Build history of the part. All positions in model axes, mm. Give positions to 0.01 mm unless a question says otherwise; leave off trailing zeros. Loops run counter-clockwise (first coordinate to the right, second up) from the corner with the lowest first, then second, coordinate; pieces in that order, holes last. Notation, with made-up numbers: M 63.25,62.5 L 100.25,62.5 A11 ccw 100.25,72.5 Z; hole C 63.5,86.5 d6. An arc over 180 degrees is marked long. Answer as a JSON object with one key per item and string values. Group by question number.
1. Drill centre lines: line 1 along X through (y, z) = (10.1, 27); line 2 along X through (y, z) = (12, 64). Where is each one in solid material? Low to high. Write a range as [from, to].
2. Slice it at B-B (y = 11.3). List the corners of the cut face in (x, z) (3 decimals).
3. Slice it at A-A (z = 22). List the corners of the cut face in (x, y), then the cut area to 3 significant figures.
4. Slice it at C-C (z = 61.5). List the corners of the cut face in (x, y), then the cut area to 4 significant figures.
5. Drop flat-ended pins along their axis: pin 1 Ø1.5 at (x, y) = (9.5, 10.5) entering from +Z; pin 2 Ø1.5 at (x, y) = (10, 10.5) entering from -Z. Give the stop position or say it passes through.
from build123d import *

# Parameters (mm, degrees)
BOX021_W     = 4.2
BOX021_H     = 6
BOX021_DEPTH = 15
BOX020_W     = 4.2
BOX020_H     = 6
BOX020_DEPTH = 15
BOX019_W     = 4.2
BOX019_H     = 6
BOX019_DEPTH = 15
BOX018_W     = 4.2
BOX018_H     = 6
BOX018_DEPTH = 15
BOX017_W     = 10
BOX017_H     = 10
BOX017_DEPTH = 32.4
BOX016_W     = 214
BOX016_H     = 3
BOX016_DEPTH = 96.05
FILLET001_R  = 6


with BuildPart() as obj1:
    # Box021 → Box021 (new body)
    with BuildSketch(Plane(origin=(211.4, 8, 15.25), x_dir=(1, 0, 0), z_dir=(0, 0, 1))):
        with Locations((2.1, 3)):
            Rectangle(BOX021_W, BOX021_H)
    extrude(amount=BOX021_DEPTH)


with BuildPart() as obj2:
    # Box020 → Box020 (new body)
    with BuildSketch(Plane(origin=(8.4, 8, 15.25), x_dir=(1, 0, 0), z_dir=(0, 0, 1))):
        with Locations((2.1, 3)):
            Rectangle(BOX020_W, BOX020_H)
    extrude(amount=BOX020_DEPTH)


with BuildPart() as obj3:
    # Box019 → Box019 (new body)
    with BuildSketch(Plane(origin=(8.4, 8, 71.75), x_dir=(1, 0, 0), z_dir=(0, 0, 1))):
        with Locations((2.1, 3)):
            Rectangle(BOX019_W, BOX019_H)
    extrude(amount=BOX019_DEPTH)


with BuildPart() as obj4:
    # Box018 → Box018 (new body)
    with BuildSketch(Plane(origin=(211.4, 8, 71.75), x_dir=(1, 0, 0), z_dir=(0, 0, 1))):
        with Locations((2.1, 3)):
            Rectangle(BOX018_W, BOX018_H)
    extrude(amount=BOX018_DEPTH)


with BuildPart() as usbopening:
    # Box017 → Box017 (new body)
    with BuildSketch(Plane(origin=(211.5, 4.5, 36.3), x_dir=(1, 0, 0), z_dir=(0, 0, 1))):
        with Locations((5, 5)):
            Rectangle(BOX017_W, BOX017_H)
    extrude(amount=BOX017_DEPTH)


with BuildPart() as cut009:
    # Box016 → Box016 (new body)
    with BuildSketch(Plane(origin=(5, 9.5, 10.475), x_dir=(1, 0, 0), z_dir=(0, 0, 1))):
        with Locations((107, 1.5)):
            Rectangle(BOX016_W, BOX016_H)
    extrude(amount=BOX016_DEPTH)

    # Fillet001
    fillet001_edges = [cut009.edges().sort_by_distance(p)[0] for p in [
        (5, 11, 106.525),
        (5, 11, 10.475),
        (219, 11, 106.525),
        (219, 11, 10.475),
    ]]
    fillet(fillet001_edges, radius=FILLET001_R)

    # Cut005: cut USBOpening
    add(usbopening.part, mode=Mode.SUBTRACT)

    # Cut006: cut obj4
    add(obj4.part, mode=Mode.SUBTRACT)

    # Cut007: cut obj3
    add(obj3.part, mode=Mode.SUBTRACT)

    # Cut008: cut obj2
    add(obj2.part, mode=Mode.SUBTRACT)

    # Cut009: cut obj1
    add(obj1.part, mode=Mode.SUBTRACT)


solid = cut009.part
Established:
{
 "1": {"line 1": "x = [5, 8.4], [12.6, 211.4], [215.6, 219]", "line 2": "x = [5, 211.5]"},
 "2": {"outline": "M 5,16.475 A6 ccw 11,10.475 L 213,10.475 A6 ccw 219,16.475 L 219,36.3 L 211.5,36.3 L 211.5,68.7 L 219,68.7 L 219,100.525 A6 ccw 213,106.525 L 11,106.525 A6 ccw 5,100.525 Z; hole M 8.4,15.25 L 12.6,15.25 L 12.6,30.25 L 8.4,30.25 Z; hole M 8.4,71.75 L 12.6,71.75 L 12.6,86.75 L 8.4,86.75 Z; hole M 211.4,15.25 L 215.6,15.25 L 215.6,30.25 L 211.4,30.25 Z; hole M 211.4,71.75 L 215.6,71.75 L 215.6,86.75 L 211.4,86.75 Z"},
 "3": {"outline": "M 5,9.5 L 8.4,9.5 L 8.4,12.5 L 5,12.5 Z; M 12.6,9.5 L 211.4,9.5 L 211.4,12.5 L 12.6,12.5 Z; M 215.6,9.5 L 219,9.5 L 219,12.5 L 215.6,12.5 Z", "area": "617 mm^2"},
 "4": {"outline": "M 5,9.5 L 211.5,9.5 L 211.5,12.5 L 5,12.5 Z", "area": "619.5 mm^2"},
 "5": {"pin 1": "stops at z = 106.48", "pin 2": "stops at z = 10.48"}
}
